For this review, use the dimensioned drawing (mm, ordinates from the lowest corner) and the shaded views. A direction names the side the tool comes from. Round coordinates to 2 decimals unless told otherwise and drop trailing zeros. Loops run counter-clockwise (first coordinate to the right, second up) from the corner with the lowest first, then second, coordinate; pieces in that order, holes last. Notation, with made-up numbers: (22.5, 63.5) - (70.5, 63.5) arc R18 ccw to (70.5, 68.5) - close; hole circle Ø3 at (-5, -5). An arc over 180 degrees is marked (long way). One line per question, with ' | ' between items. Start each with the question number.
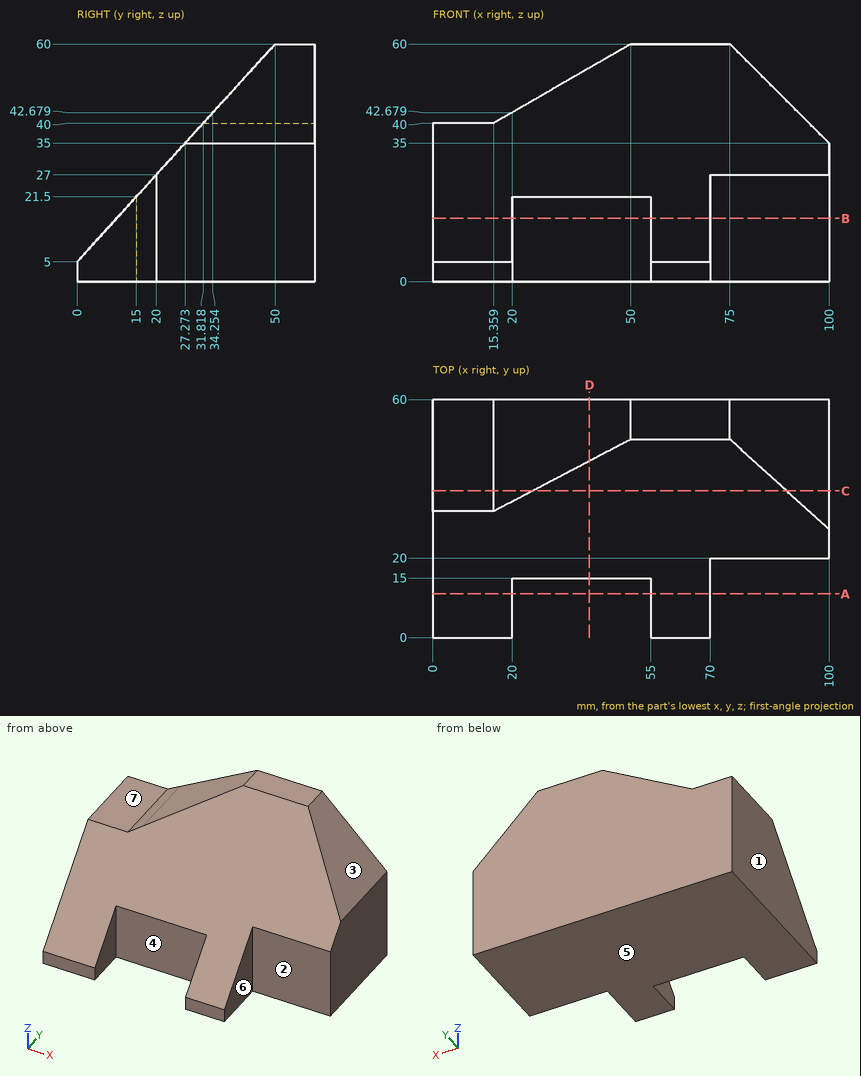
1. Take a section at C-C, the plane y = 37. Give the boundary of the cut face in (x, z), then the cut area to 3 significant figures.
2. To check wall thickness, follow line 1 along Y through (x, z) = (85, 14); line 2 along Y through (x, z) = (33, 6); line 3 along Z through (x, y) = (79, 32). State the ranges of each line that lie inside material, in increasing order.
3. Take a section at A-A, the plane y = 11. Give the boundary of the cut face in (x, z).
4. The part is to be moulded in two halves that separate along X. For the marked faces 1, 2, 3 and 4, say which applies: pulls with the +X half, pulls with the -X half, needs draft (parallel to the pull), parting line crosses it, or undercut.
5. Machinability: for the marked faces 5, 6 and 7, which of the approach directions +Z, -Z, +X, -X, +Y, -Y give a long, thin tool a straight path to every point of the face, cutting with its end or side? Answer none if there is none.
6. Take a section at D-D, the plane x = 39.5. Give the boundary of the cut face in (y, z), then the cut area to 3 significant figures.
7. Take a section at B-B, the plane z = 16. Give the boundary of the cut face in (x, y).
8. Clearance check with flat-ended pins moving along their axes: P1, Ø10, axis at y = 9.5, z = 12, coming from the +X side; P2, Ø8, axis at x = 89, z = 43, coming from the -Y side; P3, Ø4, axis at x = 66, y = 18.5, coming from the +Z side. State where each tip first meets the part, or that it passes through.
Answer list:
1) outline: (0, 0) - (100, 0) - (100, 35) - (89.3, 45.7) - (25.23, 45.7) - (15.36, 40) - (0, 40) - close | area: 4,400 mm²
2) line 1: y = 20 to 60 | line 2: y = 15 to 60 | line 3: z = 0 to 40.2
3) outline: (0, 0) - (20, 0) - (20, 17.1) - (0, 17.1) - close; (55, 0) - (70, 0) - (70, 17.1) - (55, 17.1) - close
4) face 1: pulls with the -X half | face 2: needs draft | face 3: pulls with the +X half | face 4: undercut
5) face 5: -Z, +X, -X, +Y, -Y | face 6: +Z, -Z, +X, -Y | face 7: +Z, -X, +Y, -Y
6) outline: (15, 0) - (60, 0) - (60, 53.94) - (44.49, 53.94) - (15, 21.5) - close | area: 1,950 mm²
7) outline: (0, 10) - (20, 10) - (20, 15) - (55, 15) - (55, 10) - (70, 10) - (70, 20) - (100, 20) - (100, 60) - (0, 60) - close
8) P1: stops at x = 70 | P2: stops at y = 30.91 | P3: stops at z = 27.55
